Could you check a few things on this model? Use its own coordinates, in mm. Face numbers are marked on the shaded views. A direction names the side the tool comes from. Give positions to 0.01 mm unless a question says otherwise; leave off trailing zeros. Order: outer loops, then holes, each group sorted by start corner. A loop starts at its lowest first (then second) coordinate and runs counter-clockwise, first axis right, second up. Notation, with made-up numbers: (-17, 66) -> (-4, 66) arc R23 cw to (-4, 83) -> close; hole circle Ø4 at (0.5, -35). An arc over 180 degrees is marked (long way). Write each question's results on one line, items separated by ' | '.
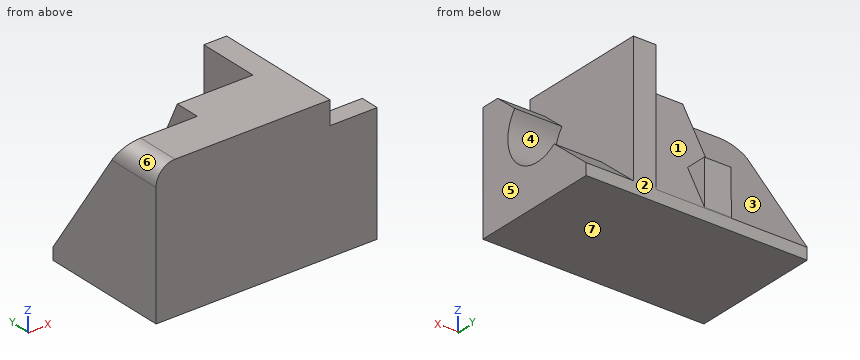
Autodesk Inventor part; units mm, degrees
ref_plane "YZ Plane" through (0, 0, 0) normal (1, 0, 0) x (0, 1, 0)
ref_plane "XZ Plane" through (0, 0, 0) normal (0, 1, 0) x (-1, 0, 0)
ref_plane "XY Plane" through (0, 0, 0) normal (0, 0, 1) x (1, 0, 0)
sketch "스케치1" plane through (0, 0, 0) normal (0, 0, 1) x (1, 0, 0)
  line L0 (18.416, -13.8824) -> (-18.416, -13.8824)
  line L1 (-18.416, -13.8824) -> (-18.416, 13.8824)
  line L2 (-18.416, 13.8824) -> (18.416, 13.8824)
  line L3 (18.416, 13.8824) -> (18.416, -13.8824)
  line L4 (18.416, -13.8824) -> (-18.416, 13.8824) construction
  line L5 (-18.416, -13.8824) -> (18.416, 13.8824) construction
  point P0 (0, 0)
extrude "돌출1" add sketch "스케치1" along normal blind 30
sketch "스케치2" plane through (18.416, -13.8824, 0) normal (1, 0, 0) x (0, 0, -1)
  line L0 (0, 27.7648) -> (0, 0)
  line L1 (0, 0) -> (-30, 0)
  line L2 (-25.0736, 0) -> (-25.0736, 4.0058)
  line L3 (-25.0736, 4.0058) -> (-21.1597, 8.5925)
  arc A0 (-21.1597, 8.5925) -> (-9.7848, 19.1723) centre (-16.0979, 14.5551) ccw
  line L4 (-9.7848, 19.1723) -> (-2.4526, 27.7648)
  line L5 (0, 27.7648) -> (-30, 27.7648)
  line L6 (0, 27.7648) -> (0, 0)
  point P0 (0, 13.8824)
extrude "돌출2" add sketch "스케치2" along normal blind 10
sketch "스케치3" plane through (-18.416, -13.8824, 0) normal (-1, 0, 0) x (0, 0, 1)
  line L0 (9.7848, 19.1723) -> (2.4526, 27.7648)
  line L1 (0, 27.7648) -> (30, 27.7648)
  line L2 (2.4526, 27.7648) -> (0, 27.7648)
  line L3 (0, 27.7648) -> (0, 6.044)
  line L4 (0, 0) -> (0, 27.7648)
  line L5 (30, 9.2244) -> (2.4526, 27.7648)
  line L6 (30, 9.2244) -> (30, 27.7648)
  point P0 (0, 13.8824)
extrude "돌출3" cut sketch "스케치3" against normal blind 16
sketch "스케치4" plane through (-2.416, -13.8824, 0) normal (-1, 0, 0) x (0, 0, 1)
  line L0 (2.4526, 27.7648) -> (30, 27.7648)
  line L1 (2.4526, 27.7648) -> (30, 14.5898)
  line L2 (30, 27.7648) -> (30, 9.2244)
  line L3 (30, 27.7648) -> (2.4526, 27.7648)
  point P0 (0, 13.8824)
extrude "돌출4" cut sketch "스케치4" against normal blind 16
sketch "스케치5" plane through (-2.416, 0.7074, 30) normal (0, 0.9021329, 0.4314583) x (1, 0, 0)
  line L0 (0, -2.315) -> (0, 30.5359)
  line L1 (5.6646, 30.341) -> (0, 30.341)
  line L2 (0, 30.341) -> (0, 19.6839)
  line L3 (0, 19.6839) -> (5.6646, 19.6839)
  line L4 (5.6646, 19.6839) -> (5.6646, 30.341)
  point P0 (2.416, 26.7588)
extrude "돌출5" add sketch "스케치5" along normal blind 5
sketch "스케치6" plane through (-2.416, -13.8824, 0) normal (-1, 0, 0) x (0, 0, 1)
  line L0 (30, 14.5898) -> (2.4526, 27.7648)
  line L1 (12.2425, 23.0826) -> (14.3998, 27.5933)
  line L2 (2.6284, 27.6807) -> (14.3998, 27.5933)
  line L3 (4.7857, 32.1914) -> (14.3998, 27.5933)
  line L4 (14.3998, 27.5933) -> (4.7857, 32.1914)
  line L5 (4.7857, 32.1914) -> (2.6284, 27.6807)
  point P0 (0, 13.8824)
extrude "돌출6" cut sketch "스케치6" against normal blind 9 contours L5 L3 L2
sketch "스케치7" plane through (-2.416, -13.8824, 0) normal (-1, 0, 0) x (0, 0, 1)
  line L0 (12.2425, 23.0826) -> (14.3998, 27.5933)
  line L1 (14.3998, 27.5933) -> (12.2425, 23.0826)
  line L2 (12.2425, 23.0826) -> (12.2425, 27.6093)
  line L3 (14.3998, 27.5933) -> (2.6284, 27.6807)
  point P0 (0, 13.8824)
extrude "돌출7" cut sketch "스케치7" against normal blind 9
fillet "모깎기1" radius 4 1 edges at (-18.416, -9.2702, 30)
properties part number "240516_3Dsketch01"
Q1. Suppose I cut it at B-B on x = 20. Please give me the cut outline in (y, z).
Here are the results:
outline: (-13.88, 0) -> (13.88, 0) -> (13.88, 2.45) -> (5.29, 9.78) arc R7.82 cw to (-5.29, 21.16) -> (-9.88, 25.07) -> (-13.88, 25.07) -> close
Q2. For the marked faces 1, 2 and 3, which set-ups out of +Z, -Z, +X, -X, +Y, -Y let a thin tool reach every point of the face, with its end or its side?
Here are the results:
face 1: +Z, +Y | face 2: +Z, -Z, +X, -X, +Y | face 3: +Z, -X, +Y
Q3. Suppose I cut it at C-C on z = 18. Please give me the cut outline in (x, y), and give its area (3 significant figures).
Here are the results:
outline: (-18.42, -13.88) -> (28.42, -13.88) -> (28.42, -6.91) -> (18.42, -6.91) -> (18.42, 13.88) -> (13.58, 13.88) -> (13.58, 6.45) -> (-2.42, 6.45) -> (-2.42, 3.42) -> (-18.42, 3.42) -> close | area: 806 mm²
Q4. I need wall thicknesses on line 1 along X through (y, z) = (3.75, 23); line 2 along X through (y, z) = (-4, 22.75); line 3 along Y through (x, z) = (22.5, 16). Which ranges of each line are inside material? Lowest first, please.
Here are the results:
line 1: x = -2.42 to 18.42 | line 2: x = -18.42 to 18.42 | line 3: y = -13.88 to -7.15
Q5. Thinking about a two-plate mould opening in Z: for the marked faces 4, 5, 6 and 7, which applies, +Z half, -Z half, draft (parallel to the pull), parting line (faces both ways), or undercut?
Here are the results:
face 4: undercut | face 5: draft | face 6: +Z half | face 7: -Z half
Q6. Suppose I cut it at D-D on y = 8.5. Please give me the cut outline in (x, z), and give its area (3 significant figures).
Here are the results:
outline: (-18.42, 0) -> (28.42, 0) -> (28.42, 7.05) -> (18.42, 7.05) -> (18.42, 30) -> (13.58, 30) -> (13.58, 13.71) -> (-2.42, 13.71) -> (-2.42, 10.45) -> (-18.42, 10.45) -> close | area: 602 mm²
Q7. I'm going to push flat-ended pins straight in: pin 1 Ø2 at (x, z) = (3, 19.5) entering from +Y; pin 2 Ø4 at (y, z) = (8.5, 17) entering from +X; pin 3 Ø2.5 at (x, y) = (1.5, 11) entering from +Z. Where does each tip first touch, or does it pass through?
Here are the results:
pin 1: stops at y = 6.21 | pin 2: stops at x = 18.42 | pin 3: stops at z = 12.24
Q8. Suppose I cut it at A-A on y = -6.5. Please give me the cut outline in (x, z).
Here are the results:
outline: (-18.42, 0) -> (28.42, 0) -> (28.42, 12.98) -> (18.42, 12.98) -> (18.42, 19.22) -> (28.42, 19.22) -> (28.42, 22.19) -> (18.42, 22.19) -> (18.42, 30) -> (-14.42, 30) arc R4 ccw to (-18.42, 26) -> close
